Could you check a few things on this model? Use its own coordinates, in mm. A direction names the side the tool comes from. Give positions to 0.01 mm unless a question says otherwise; leave off trailing zeros. Loops run counter-clockwise (first coordinate to the right, second up) from the corner with the lowest first, then second, coordinate; pieces in that order, holes last.
1. For P1, Ø3, axis at y = 20, z = 40, coming from the -X side; P2, Ø6.5, axis at y = -20, z = -40, coming from the +X side; P3, Ø8, axis at x = 107, z = -16.5, coming from the -Y side; P4, Ø3, axis at x = 71.5, y = 0, coming from the +Z side, each with a flat end and sliding along its axis, tell me the tip position at first contact or that it passes through.
2. Imagine slicing it at D-D (z = -27). List the corners of the cut face in (x, y) for me, plus the area to 3 significant figures.
3. Imagine slicing it at C-C (z = 0). List the corners of the cut face in (x, y) for me.
4. Thinking about a two-plate mould opening in Y: for faces 4 (the flat face through (86, 3, -1)), 5 (the cylindrical face through (2.54, 22.11, 38.66)), 6 (the cylindrical face through (111.298, 0.042, -2.506)), which applies, +Y half, -Y half, draft (parallel to the pull), parting line (faces both ways), or undercut?
5. Imagine slicing it at A-A (y = -20). List the corners of the cut face in (x, z) for me, plus the area to 3 significant figures.
6. I need wall thicknesses on line 1 along Y through (x, z) = (1.3, -40); line 2 along X through (y, z) = (1.35, 0); line 3 along X through (y, z) = (25.5, -45.5). Which ranges of each line are inside material? Lowest first, please.
7. Imagine slicing it at B-B (x = 109). List the corners of the cut face in (y, z) for me.
8. For faces 1 (the flat face through (86, -3, -1)), 2 (the cylindrical face through (2.535, -19.249, -42.385)), 3 (the flat face through (84, 0, -45)), which set-ups out of +Z, -Z, +X, -X, +Y, -Y let a thin tool reach every point of the face, with its end or its side?
```python
from build123d import *

# Parameters (mm, degrees)
SKETCH_1_W          = 100
SKETCH_1_H          = 60
EXTRUDE_1_DEPTH     = 5
CUT_EXTRUDE_1_REACH = 7
SKETCH_2_R          = 2.5
EXTRUDE_2_DEPTH     = 3
CUT_EXTRUDE_2_REACH = 35
SKETCH_4_R          = 3.4


with BuildPart() as part:
    # 스케치1 → 보스-돌출1 (new body)
    with BuildSketch(Plane(origin=(0, 0, 0), x_dir=(0, 0, -1), z_dir=(1, 0, 0))):
        Rectangle(SKETCH_1_W, SKETCH_1_H)
    extrude(amount=EXTRUDE_1_DEPTH)

    # 스케치2 → 컷-돌출1 (cut, up to next)
    with BuildSketch(Plane(origin=(5, 0, 0), x_dir=(0, 0, -1), z_dir=(1, 0, 0)), mode=Mode.PRIVATE) as cut_extrude_1_sk1:
        with Locations((-40, 20)):
            Circle(SKETCH_2_R)
    cut_extrude_1_tool1 = extrude(cut_extrude_1_sk1.sketch, amount=-CUT_EXTRUDE_1_REACH, mode=Mode.PRIVATE) & part.part
    add(cut_extrude_1_tool1.solids().sort_by_distance((5, 20, 40))[0], mode=Mode.SUBTRACT)
    # 스케치2 → 컷-돌출1 (cut, up to next)
    with BuildSketch(Plane(origin=(5, 0, 0), x_dir=(0, 0, -1), z_dir=(1, 0, 0)), mode=Mode.PRIVATE) as cut_extrude_1_sk2:
        with Locations((-40, -20)):
            Circle(SKETCH_2_R)
    cut_extrude_1_tool2 = extrude(cut_extrude_1_sk2.sketch, amount=-CUT_EXTRUDE_1_REACH, mode=Mode.PRIVATE) & part.part
    add(cut_extrude_1_tool2.solids().sort_by_distance((5, -20, 40))[0], mode=Mode.SUBTRACT)
    # 스케치2 → 컷-돌출1 (cut, up to next)
    with BuildSketch(Plane(origin=(5, 0, 0), x_dir=(0, 0, -1), z_dir=(1, 0, 0)), mode=Mode.PRIVATE) as cut_extrude_1_sk3:
        with Locations((40, -20)):
            Circle(SKETCH_2_R)
    cut_extrude_1_tool3 = extrude(cut_extrude_1_sk3.sketch, amount=-CUT_EXTRUDE_1_REACH, mode=Mode.PRIVATE) & part.part
    add(cut_extrude_1_tool3.solids().sort_by_distance((5, -20, -40))[0], mode=Mode.SUBTRACT)
    # 스케치2 → 컷-돌출1 (cut, up to next)
    with BuildSketch(Plane(origin=(5, 0, 0), x_dir=(0, 0, -1), z_dir=(1, 0, 0)), mode=Mode.PRIVATE) as cut_extrude_1_sk4:
        with Locations((40, 20)):
            Circle(SKETCH_2_R)
    cut_extrude_1_tool4 = extrude(cut_extrude_1_sk4.sketch, amount=-CUT_EXTRUDE_1_REACH, mode=Mode.PRIVATE) & part.part
    add(cut_extrude_1_tool4.solids().sort_by_distance((5, 20, -40))[0], mode=Mode.SUBTRACT)

    # 스케치3 → 보스-돌출2 (add, symmetric)
    with BuildSketch(Plane(origin=(0, 0, 0), x_dir=(1, 0, 0), z_dir=(0, 1, 0))):
        Polygon((170, 35), (160, 45), (5, 45), (5, -45), (160, -45), (170, -35), align=None)
    extrude(amount=EXTRUDE_2_DEPTH, both=True)

    # 스케치4 → 컷-돌출2 (cut, up to next)
    with BuildSketch(Plane(origin=(0, 3, 0), x_dir=(1, 0, 0), z_dir=(0, 1, 0)), mode=Mode.PRIVATE) as cut_extrude_2_sk1:
        with Locations(Location((57, 0, 0), (0, 0, 270))):  # turned: the seam where the file's is
            Circle(SKETCH_4_R)
    cut_extrude_2_tool1 = extrude(cut_extrude_2_sk1.sketch, amount=-CUT_EXTRUDE_2_REACH, mode=Mode.PRIVATE) & part.part
    add(cut_extrude_2_tool1.solids().sort_by_distance((57, 3, 0))[0], mode=Mode.SUBTRACT)
    # 스케치4 → 컷-돌출2 (cut, up to next)
    with BuildSketch(Plane(origin=(0, 3, 0), x_dir=(1, 0, 0), z_dir=(0, 1, 0)), mode=Mode.PRIVATE) as cut_extrude_2_sk2:
        with Locations(Location((109, 0, 0), (0, 0, 270))):  # turned: the seam where the file's is
            Circle(SKETCH_4_R)
    cut_extrude_2_tool2 = extrude(cut_extrude_2_sk2.sketch, amount=-CUT_EXTRUDE_2_REACH, mode=Mode.PRIVATE) & part.part
    add(cut_extrude_2_tool2.solids().sort_by_distance((109, 3, 0))[0], mode=Mode.SUBTRACT)
    # 스케치4 → 컷-돌출2 (cut, up to next)
    with BuildSketch(Plane(origin=(0, 3, 0), x_dir=(1, 0, 0), z_dir=(0, 1, 0)), mode=Mode.PRIVATE) as cut_extrude_2_sk3:
        with Locations(Location((161, 0, 0), (0, 0, 270))):  # turned: the seam where the file's is
            Circle(SKETCH_4_R)
    cut_extrude_2_tool3 = extrude(cut_extrude_2_sk3.sketch, amount=-CUT_EXTRUDE_2_REACH, mode=Mode.PRIVATE) & part.part
    add(cut_extrude_2_tool3.solids().sort_by_distance((161, 3, 0))[0], mode=Mode.SUBTRACT)


solid = part.part
```
Derived:
1. P1: passes through
1. P2: stops at x = 5
1. P3: stops at y = -3
1. P4: stops at z = 45
2. outline: (0, -30) - (5, -30) - (5, -3) - (170, -3) - (170, 3) - (5, 3) - (5, 30) - (0, 30) - close
2. area: 1,290 mm2
3. outline: (0, -30) - (5, -30) - (5, -3) - (53.6, -3) - (53.6, 3) - (5, 3) - (5, 30) - (0, 30) - close; (60.4, -3) - (105.6, -3) - (105.6, 3) - (60.4, 3) - close; (112.4, -3) - (157.6, -3) - (157.6, 3) - (112.4, 3) - close; (164.4, -3) - (170, -3) - (170, 3) - (164.4, 3) - close
4. face 4: +Y half
4. face 5: undercut
4. face 6: draft
5. outline: (0, -50) - (5, -50) - (5, -42.5) - (0, -42.5) - close; (0, -37.5) - (5, -37.5) - (5, 37.5) - (0, 37.5) - close; (0, 42.5) - (5, 42.5) - (5, 50) - (0, 50) - close
5. area: 450 mm2
6. line 1: y = -30 to -22.5, -17.5 to 17.5, 22.5 to 30
6. line 2: x = 0 to 53.6, 60.4 to 105.6, 112.4 to 157.6, 164.4 to 170
6. line 3: x = 0 to 5
7. outline: (-3, -45) - (3, -45) - (3, -3.4) - (-3, -3.4) - close; (-3, 3.4) - (3, 3.4) - (3, 45) - (-3, 45) - close
8. face 1: +Z, -Z, +X, -Y
8. face 2: +X, -X
8. face 3: -Z, +X, +Y, -Y
